Part model, mm, in its own coordinate system. A direction names the side the tool comes from. Round coordinates to 2 decimals unless told otherwise and drop trailing zeros. Loops run counter-clockwise (first coordinate to the right, second up) from the corner with the lowest first, then second, coordinate; pieces in that order, holes last. Notation, with made-up numbers: M 82,82.5 L 108,82.5 A15 ccw 108,101.5 Z; hole C -22,53.5 d8. An arc over 180 degrees is marked long. Put each result on its own line as item: value. Start each with the question number.
1) Probe line 1 along X through (y, z) = (10, 20); line 2 along Y through (x, z) = (45, 1); line 3 along Z through (x, y) = (12, 6.5). List the from-to ranges inside material, lowest first.
2) Slice it at A-A on y = 23. Give the cut face in (x, z), then the cut area to 3 significant figures.
3) Drop flat-ended pins along their axis: pin 1 Ø5 at (y, z) = (25, 9) entering from +X; pin 2 Ø1 at (y, z) = (26, 8.5) entering from +X; pin 3 Ø2 at (x, y) = (45.5, 5.5) entering from -Z. Give the stop position or say it passes through.
4) Which spindle directions (+Z, -Z, +X, -X, +Y, -Y) get a long thin tool onto all of the face, cutting with end or side? Do faces 1 (the flat face through (37.1, 12.5, 21.4)), 2 (the flat face through (4, 7, 24)), 3 (the flat face through (42, 9, 2)), 4 (the flat face through (47, 3.4, 15.2)). Say none if no direction does.
5) Pull direction X, two halves, no side cores. Call faces 5 (the cylindrical face through (0.57, 14.4, 21.45)), 6 (the flat face through (19, 15, 1)), 7 (the flat face through (16.8, 15, 35.3)): +X half, -X half, draft (parallel to the pull), parting line (faces both ways), or undercut.
```python
from build123d import *

# Parameters (mm, degrees)
BOSS_EXTRU_1_DEPTH      = 43.5
ESQUISSE2_W             = 2
ESQUISSE2_H             = 15
BOSS_EXTRU_2_DEPTH      = 49
ESQUISSE4_W             = 2
ESQUISSE4_H             = 8.9
BOSS_EXTRU_3_DEPTH      = 39
ESQUISSE5_W             = 5
ESQUISSE5_H             = 5
BOSS_EXTRU_4_DEPTH      = 4.5
CONG_1_R                = 2
CONG_2_R                = 2
CONG_5_R                = 2
ESQUISSE6_R             = 12.5
ENL_V_MAT_EXTRU_1_DEPTH = 2.5
CHANFREIN1_SIZE         = 2
ESQUISSE7_R             = 1.8
ENL_V_MAT_EXTRU_2_DEPTH = 3.8
CHANFREIN3_SIZE         = 0.5
ESQUISSE8_R             = 20
ESQUISSE8_R_2           = 17.1
BOSS_EXTRU_5_DEPTH      = 14
CONG_6_R                = 2
CONG_7_R                = 2
CHANFREIN4_SIZE         = 0.5


with BuildPart() as part:
    # Esquisse1 → Boss.-Extru.1 (new body)
    with BuildSketch(Plane.XY):
        Polygon((6, 0), (0, 0), (0, 15), (49, 15), (49, 0), (43, 0), (47, 3), (47, 12.5), (2, 12.5), (2, 3), align=None)
    extrude(amount=BOSS_EXTRU_1_DEPTH)

    # Esquisse2 → Boss.-Extru.2 (add)
    with BuildSketch(Plane.ZY):
        with Locations((44.5, 7.5)):
            Rectangle(ESQUISSE2_W, ESQUISSE2_H)
    extrude(amount=-BOSS_EXTRU_2_DEPTH)

    # Esquisse4 → Boss.-Extru.3 (add)
    with BuildSketch(Plane(origin=(0, 0, 43.5), x_dir=(-1, 0, 0), z_dir=(0, 0, -1))):
        with Locations((-46, 8.05)):
            Rectangle(ESQUISSE4_W, ESQUISSE4_H)
        with Locations((-3, 8.05)):
            Rectangle(ESQUISSE4_W, ESQUISSE4_H)
    extrude(amount=BOSS_EXTRU_3_DEPTH)

    # Esquisse5 → Boss.-Extru.4 (add)
    with BuildSketch(Plane(origin=(0, 0, 4.5), x_dir=(-1, 0, 0), z_dir=(0, 0, -1))):
        with Locations((-44.5, 10)):
            Rectangle(ESQUISSE5_W, ESQUISSE5_H)
        with Locations((-4.5, 10)):
            Rectangle(ESQUISSE5_W, ESQUISSE5_H)
    extrude(amount=BOSS_EXTRU_4_DEPTH)

    # Congé1
    cong_1_edges = [part.edges().sort_by_distance(p)[0] for p in [
        (45, 12.5, 24),
        (4, 12.5, 24),
    ]]
    fillet(cong_1_edges, radius=CONG_1_R)

    # Congé2
    cong_2_edges = [part.edges().sort_by_distance(p)[0] for p in [
        (42, 12.5, 2.25),
        (7, 12.5, 2.25),
    ]]
    fillet(cong_2_edges, radius=CONG_2_R)

    # Congé5
    cong_5_edges = [part.edges().sort_by_distance(p)[0] for p in [
        (0, 15, 22.75),
        (49, 15, 22.75),
        (49, 7.5, 45.5),
        (24.5, 15, 45.5),
        (0, 7.5, 45.5),
    ]]
    fillet(cong_5_edges, radius=CONG_5_R)

    # Esquisse6 → Enlèv. mat.-Extru.1 (cut)
    with BuildSketch(Plane(origin=(0, 15, 0), x_dir=(1, 0, 0), z_dir=(0, 1, 0))):
        with Locations(Location((24.5, -22.75, 0), (0, 0, 270))):
            Circle(ESQUISSE6_R)
    extrude(amount=-ENL_V_MAT_EXTRU_1_DEPTH, mode=Mode.SUBTRACT)

    # Chanfrein1
    chanfrein1_edges = [part.edges().sort_by_distance(p)[0] for p in [
        (24.5, 15, 10.25),
    ]]
    chamfer(chanfrein1_edges, length=CHANFREIN1_SIZE)

    # Esquisse7 → Enlèv. mat.-Extru.2 (cut)
    with BuildSketch(Plane(origin=(0, 0, 0), x_dir=(-1, 0, 0), z_dir=(0, 0, -1))):
        with Locations((-45.5, 11)):
            Circle(ESQUISSE7_R)
        with Locations((-3.5, 11)):
            Circle(ESQUISSE7_R)
    extrude(amount=-ENL_V_MAT_EXTRU_2_DEPTH, mode=Mode.SUBTRACT)

    # Chanfrein3
    chanfrein3_edges = [part.edges().sort_by_distance(p)[0] for p in [
        (47.3, 11, 0),
        (5.3, 11, 0),
    ]]
    chamfer(chanfrein3_edges, length=CHANFREIN3_SIZE)

    # Esquisse8 → Boss.-Extru.5 (add)
    with BuildSketch(Plane(origin=(0, 15, 0), x_dir=(1, 0, 0), z_dir=(0, 1, 0))):
        with Locations(Location((24.5, -22.75, 0), (0, 0, 90))):
            Circle(ESQUISSE8_R)
        with Locations(Location((24.5, -22.75, 0), (0, 0, 270))):
            Circle(ESQUISSE8_R_2, mode=Mode.SUBTRACT)
    extrude(amount=BOSS_EXTRU_5_DEPTH)

    # Congé6
    cong_6_edges = [part.edges().sort_by_distance(p)[0] for p in [
        (24.5, 15, 42.75),
    ]]
    fillet(cong_6_edges, radius=CONG_6_R)

    # Congé7
    cong_7_edges = [part.edges().sort_by_distance(p)[0] for p in [
        (24.5, 29, 42.75),
    ]]
    fillet(cong_7_edges, radius=CONG_7_R)

    # Chanfrein4
    chanfrein4_edges = [part.edges().sort_by_distance(p)[0] for p in [
        (24.5, 29, 5.65),
    ]]
    chamfer(chanfrein4_edges, length=CHANFREIN4_SIZE)


solid = part.part
```
Recorded:
1. line 1: x = 0 to 4, 45 to 49
1. line 2: y = 0 to 1.5, 7.5 to 9.27, 12.73 to 15
1. line 3: z = 43.5 to 45.5
2. outline: C 24.5,22.75 d40; hole C 24.5,22.75 d34.2
2. area: 338 mm2
3. pin 1: stops at x = 41.04
3. pin 2: stops at x = 39.02
3. pin 3: stops at z = 4.5
4. face 1: -Y
4. face 2: none
4. face 3: -Z, -Y
4. face 4: -Z
5. face 5: -X half
5. face 6: draft
5. face 7: undercut
